```python
from build123d import *

# Parameters (mm, degrees)
F1_DEPTH = 6.35
F2_R     = 15.24
F2_R_2   = 12.7
F3_DEPTH = 6.35
F4_R     = 1.27
F5_DEPTH = 6.35


with BuildPart() as f1:
    # F0 (on Front) → F1 (new body)
    with BuildSketch(Plane.XZ):
        Polygon((7.3323484187, 12.7), (-7.3323484187, 12.7), (0, 0), align=None)
    extrude(amount=F1_DEPTH)



with BuildPart() as f1b:
    # F0 (on Front) → F1, piece 2 (new body)
    with BuildSketch(Plane.XZ):
        Polygon((0, 0), (-14.6646968374, 0), (-7.3323484187, -12.7), align=None)
    extrude(amount=F1_DEPTH)


with BuildPart() as f1c:
    # F0 (on Front) → F1, piece 3 (new body)
    with BuildSketch(Plane.XZ):
        Polygon((14.6646968374, 0), (0, 0), (7.3323484187, -12.7), align=None)
    extrude(amount=F1_DEPTH)


with BuildPart() as f1_1:
    add(f1.part)

    add(f1b.part)  # F3 merges F1b

    add(f1c.part)  # F3 merges F1c
    # F2 (on Front) → F3 (join)
    with BuildSketch(Plane.XZ):
        Circle(F2_R)
        Circle(F2_R_2, mode=Mode.SUBTRACT)
    extrude(amount=F3_DEPTH)

    # F4 (on Front) → F5 (join)
    with BuildSketch(Plane.XZ):
        Circle(F4_R)
    extrude(amount=F5_DEPTH)


solid = f1_1.part
```
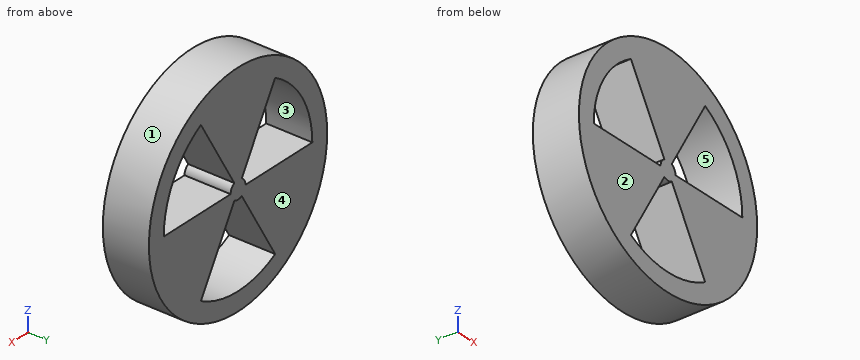
Source: CAD feature listing. Evaluate the final solid. Frame: model axes, mm. Face numbers are marked on the shaded views. A direction names the side the tool comes from. Round coordinates to 2 decimals unless told otherwise and drop trailing zeros. Loops run counter-clockwise (first coordinate to the right, second up) from the corner with the lowest first, then second, coordinate; pieces in that order, holes last. Notation, with made-up numbers: M -27.5,54.25 L 1.5,54.25 A22 ccw 1.5,79.25 Z; hole C 24.25,-3 d4. An arc over 180 degrees is marked long. Use a Markdown table: item, result. Add a question column.
1. Set-up query: the marked faces 4 and 5. Return all of +Z, -Z, +X, -X, +Y, -Y with unobstructed straight access to the full face (end or side cutting, diameter ignored); none if empty.
2. Cut plane D-D, the plane x = 8. Output: boundary loops of the cut face in (y, z).
3. Cut plane B-B, the plane x = 2. Output: boundary loops of the cut face in (y, z).
4. Ray query, line 1 along Z through (x, y) = (4, -2.75); line 2 along X through (y, z) = (-2.25, 8); line 3 along Z through (x, y) = (-1, -0.25). Return the intervals inside material, ascending. Write a range as [from, to].
5. Pull-direction query (X, two-part tool) for the marked faces 1, 2 and 3; classes: +X half, -X half, draft (parallel to the pull), parting line (faces both ways), or undercut.
6. Cut plane A-A, the plane y = -4.5. Output: boundary loops of the cut face in (x, z) (3 decimals), and give its area (3 significant figures).
7. Contact query for flat-ended pins moving along their axis: pin 1 (1.9 mm diameter, centred on x = -8.5, y = -4.5, fed in from +Z); pin 2 (3 mm diameter, centred on y = -1, z = 3.5, fed in from +X); pin 3 (1.5 mm diameter, centred on x = 10, z = 4, fed in from +Y). Output: stop coordinate, or through.
8. Cut plane C-C, the plane z = -4. Output: boundary loops of the cut face in (x, y).
Solution:
| question | item | result |
|---|---|---|
| 1 | face 4 | +Z, -Z, +X, -X, +Y |
| 1 | face 5 | +Y, -Y |
| 2 | outline | M -6.35,-12.97 L 0,-12.97 L 0,0 L -6.35,0 Z; M -6.35,9.86 L 0,9.86 L 0,12.97 L -6.35,12.97 Z |
| 3 | outline | M -6.35,-15.11 L 0,-15.11 L 0,-12.54 L -6.35,-12.54 Z; M -6.35,-3.46 L 0,-3.46 L 0,0 L -6.35,0 Z; M -6.35,3.46 L 0,3.46 L 0,15.11 L -6.35,15.11 Z |
| 4 | line 1 | z = [-14.71, -12.05], [-6.93, 0], [6.93, 14.71] |
| 4 | line 2 | x = [-12.97, -9.86], [-4.62, 4.62], [9.86, 12.97] |
| 4 | line 3 | z = [-15.21, -12.66], [-1.73, 0.78], [1.73, 15.21] |
| 5 | face 1 | parting line |
| 5 | face 2 | draft |
| 5 | face 3 | undercut |
| 6 | outline | C 0,0 d30.48; hole M -12.7,0 L -1.27,0 A1.27 cw -0.635,1.1 L -6.35,10.999 A12.7 ccw Z; hole M -6.35,-10.999 A12.7 ccw 6.35,-10.999 L 0.635,-1.1 A1.27 cw -0.635,-1.1 Z; hole M 0.635,1.1 A1.27 cw 1.27,0 L 12.7,0 A12.7 ccw 6.35,10.999 Z |
| 6 | area | 479 mm2 |
| 7 | pin 1 | stops at z = 13.24 |
| 7 | pin 2 | stops at x = 15.11 |
| 7 | pin 3 | passes through |
| 8 | outline | M -14.71,-6.35 L -2.31,-6.35 L -2.31,0 L -14.71,0 Z; M 2.31,-6.35 L 14.71,-6.35 L 14.71,0 L 2.31,0 Z |
